Part model, mm, in its own coordinate system. A direction names the side the tool comes from. Round coordinates to 2 decimals unless told otherwise and drop trailing zeros. Write each loop counter-clockwise with the first axis right and the second up, starting at its lowest first coordinate (ties: lowest second). Pieces come first, ordered by that corner, then holes. Notation, with made-up numbers: (71, 82.25) -> (112, 82.25) arc R15 ccw to (112, 106.25) -> close; hole circle Ø3 at (-10.75, -29.75). An arc over 180 degrees is marked (long way). Return JSON: item names as keys, results as strings. Group by question number.
(1) Tool access for faces 4 (the cylindrical face through (-14.12, -36.76, -44.83)), 5 (the cylindrical face through (-42.225, 22.187, 28.466)): list every direction of +Z, -Z, +X, -X, +Y, -Y with a clear straight run to the whole face (end or side of a thin tool).
(2) Drill centre lines: L1, parallel to X at y = 24, z = 0; L2, parallel to X at y = -19.75, z = 0; L3, parallel to Z at x = -1.5, y = -13.5. Where is each one in solid material? Low to high. Write a range as from..to.
(3) Mould opens along Y. For faces 1 (the flat face through (-1, 37.75, -27)), 2 (the cylindrical face through (-1.055, 27.736, 23.977)), 3 (the flat face through (23, 28.75, -8)) say: +Y half, -Y half, draft (parallel to the pull), parting line (faces both ways), or undercut.
(4) Saw through at B-B (y = -32). List the corners of the cut face in (x, z).
(5) Saw through at A-A (y = 15.5). List the corners of the cut face in (x, z), plus the area to 3 significant figures.
(6) Drop flat-ended pins along their axis: pin 1 Ø12 at (y, z) = (1.5, -6) entering from -X; pin 2 Ø1.5 at (x, y) = (21.5, -20.5) entering from +Z; pin 3 Ø1 at (y, z) = (-14.5, -10.5) entering from -X. Give the stop position or say it passes through.
from build123d import *

# Parameters (mm, degrees)
CUT_EXTRUDE5_START = -2.5
SKETCH3_R          = 2
CUT_EXTRUDE5_DEPTH = 50


with BuildPart() as part:
    # Sketch2 → Revolve1 (revolve)
    with BuildSketch(Plane(origin=(0, 0, 0), x_dir=(0, 0, -1), z_dir=(1, 0, 0))):
        Polygon((47, -37.75), (62.5, -37.75), (62.5, 37.75), (24, 37.75), (24, 35.75), (26, 35.75), (26, 28.75), (24, 28.75), (24, 26.75), (42.5, 26.75), (42.5, 17.75), (53, 17.75), (53, -15.75), (47, -15.75), (47, -25.75), (50, -25.75), (50, -35.75), (47, -35.75), align=None)
    revolve(axis=Axis((0, -15.437269333, 0), (0, 1, 0)))

    # Sketch3 → Cut-Extrude5 (cut)
    with BuildSketch(Plane.XZ.offset(25.75).offset(CUT_EXTRUDE5_START)):
        with Locations(Location((-47.552825815, 15.450849719, 0), (0, 0, 270))):
            Circle(SKETCH3_R)
        with Locations(Location((-40.450849719, 29.389262615, 0), (0, 0, 270))):
            Circle(SKETCH3_R)
        with Locations(Location((-29.389262615, 40.450849719, 0), (0, 0, 270))):
            Circle(SKETCH3_R)
        with Locations(Location((-15.450849719, 47.552825815, 0), (0, 0, 270))):
            Circle(SKETCH3_R)
        with Locations(Location((0, 50, 0), (0, 0, 270))):
            Circle(SKETCH3_R)
        with Locations(Location((15.450849719, 47.552825815, 0), (0, 0, 270))):
            Circle(SKETCH3_R)
        with Locations(Location((29.389262615, 40.450849719, 0), (0, 0, 270))):
            Circle(SKETCH3_R)
        with Locations(Location((40.450849719, 29.389262615, 0), (0, 0, 270))):
            Circle(SKETCH3_R)
        with Locations(Location((47.552825815, 15.450849719, 0), (0, 0, 270))):
            Circle(SKETCH3_R)
        with Locations(Location((50, 0, 0), (0, 0, 270))):
            Circle(SKETCH3_R)
        with Locations(Location((47.552825815, -15.450849719, 0), (0, 0, 270))):
            Circle(SKETCH3_R)
        with Locations(Location((40.450849719, -29.389262615, 0), (0, 0, 270))):
            Circle(SKETCH3_R)
        with Locations(Location((29.389262615, -40.450849719, 0), (0, 0, 270))):
            Circle(SKETCH3_R)
        with Locations(Location((15.450849719, -47.552825815, 0), (0, 0, 270))):
            Circle(SKETCH3_R)
        with Locations(Location((0, -50, 0), (0, 0, 270))):
            Circle(SKETCH3_R)
        with Locations(Location((-15.450849719, -47.552825815, 0), (0, 0, 270))):
            Circle(SKETCH3_R)
        with Locations(Location((-29.389262615, -40.450849719, 0), (0, 0, 270))):
            Circle(SKETCH3_R)
        with Locations(Location((-40.450849719, -29.389262615, 0), (0, 0, 270))):
            Circle(SKETCH3_R)
        with Locations(Location((-47.552825815, -15.450849719, 0), (0, 0, 270))):
            Circle(SKETCH3_R)
        with Locations(Location((-50, 0, 0), (0, 0, 270))):
            Circle(SKETCH3_R)
    extrude(amount=-CUT_EXTRUDE5_DEPTH, mode=Mode.SUBTRACT)


solid = part.part
Computed values:
{
 "1": {"face 4": "-Y", "face 5": "none"},
 "2": {"L1": "-62.5..-52, -48..-42.5, 42.5..48, 52..62.5", "L2": "-62.5..-52, -48..-47, 47..48, 52..62.5", "L3": "-62.48..-52.98, 52.98..62.48"},
 "3": {"face 1": "+Y half", "face 2": "draft", "face 3": "undercut"},
 "4": {"outline": "circle Ø125 at (0, 0); hole circle Ø100 at (0, 0)"},
 "5": {"outline": "circle Ø125 at (0, 0); hole circle Ø106 at (0, 0)", "area": "3,450 mm2"},
 "6": {"pin 1": "x = -62.5", "pin 2": "z = 58.95", "pin 3": "x = -61.69"}
}
